Input: part model. Units: mm. Frame: model coordinates. A direction names the side the tool comes from. Coordinates: 2 decimals unless noted, no trailing zeros. Write each loop counter-clockwise with the first axis right and the second up, starting at its lowest first coordinate (ties: lowest second). Pieces come first, ordered by that corner, then holes. Notation, with made-up numbers: (66.5, -24.75) - (125.5, -24.75) arc R32 ccw to (125.5, 3.25) - close; hole circle Ø1 at (16, -32.5). An arc over 180 degrees is marked (long way). Use a Markdown table: item, result. Add a question column.
Q1. Material intervals for probe 1 along Y at (x, z) = (-8, -161.5) (3 decimals); probe 2 along X at (y, z) = (4.5, -37.5) (3 decimals); probe 3 along Y at (x, z) = (24.25, 190.5) (3 decimals), sorted ascending. Write a range as from..to.
Q2. Mould query, pull axis X, two halves, no side actions, for faces 1 (the face through (0, -9.525, -5)), 2 (the face through (-25.4, 0, -5)), 3 (the face through (0, 10, 330.2)). Classes: released by +X, released by -X, zero draft, split by the parting line, or undercut.
Q3. Set-up query: faces 4 (the face through (0, -12.7, -5)), 5 (the face through (-23.79, 1.907, -152.107)), 6 (the face through (22.225, 0, -5)). Return all of +Z, -Z, +X, -X, +Y, -Y with unobstructed straight access to the full face (end or side cutting, diameter ignored); none if empty.
Q4. Section query A-A (z = 1.5). Return the cut outline in (x, y) (3 decimals).
Q5. Pin query (flat end, axial travel): P1, Ø5.5, axis at y = 0, z = -215.9, coming from the -X side. Return the tip coordinate at first contact, or that it passes through.
Q6. Section query B-B (z = 120.65). Return the cut outline in (x, y) (3 decimals).
from build123d import *

# Parameters (mm, degrees)
BOSS_EXTRUDE1_DEPTH              = 330.2
BOSS_EXTRUDE1_DEPTH_BACK         = 330.2
SKETCH3_W                        = 50.8
SKETCH3_H                        = 25.4
SKETCH3_W_2                      = 44.45
SKETCH3_H_2                      = 19.05
F_1_4_0_25_DIAMETER_HOLE3_D      = 6.35
F_1_4_0_25_DIAMETER_HOLE4_D      = 6.35
F_1_4_0_25_DIAMETER_HOLE5_D      = 6.35
F_1_4_0_25_DIAMETER_HOLE6_D      = 6.35
F_1_4_0_25_DIAMETER_HOLE7_D      = 6.35
F_1_4_0_25_DIAMETER_HOLE8_D      = 6.35
F_13_64_0_20313_DIAMETER_HOLE1_D = 5.159502
F_1_2_0_5_DIAMETER_HOLE1_D       = 12.7
F_1_2_0_5_DIAMETER_HOLE1_DEPTH   = 6.35
F_1_2_0_5_DIAMETER_HOLE1_TIP     = 3.815464931


with BuildPart() as part:
    # Sketch3 → Boss-Extrude1 (new, two sides: drawn at the far end of the back side and taken through both)
    with BuildSketch(Plane.XY.offset(-BOSS_EXTRUDE1_DEPTH_BACK)):
        Rectangle(SKETCH3_W, SKETCH3_H)
        Rectangle(SKETCH3_W_2, SKETCH3_H_2, mode=Mode.SUBTRACT)
    extrude(amount=BOSS_EXTRUDE1_DEPTH + BOSS_EXTRUDE1_DEPTH_BACK)

    # 1/4 (0.25) Diameter Hole3 (through all)
    with Locations(Plane.ZY.offset(25.4)):
        with Locations((-317.5, 0)):
            Hole(F_1_4_0_25_DIAMETER_HOLE3_D / 2)

    # 1/4 (0.25) Diameter Hole4 (through all)
    with Locations(Plane.ZY.offset(25.4)):
        with Locations((292.1, 0), (317.5, 0)):
            Hole(F_1_4_0_25_DIAMETER_HOLE4_D / 2)

    # 1/4 (0.25) Diameter Hole5 (through all)
    with Locations(Plane(origin=(25.4, 0, 0), x_dir=(0, 0, -1), z_dir=(1, 0, 0))):
        with Locations((292.1, 0), (266.7, 0)):
            Hole(F_1_4_0_25_DIAMETER_HOLE5_D / 2)

    # 1/4 (0.25) Diameter Hole6 (through all)
    with Locations(Plane(origin=(25.4, 0, 0), x_dir=(0, 0, -1), z_dir=(1, 0, 0))):
        with Locations((215.9, 0), (241.3, 0)):
            Hole(F_1_4_0_25_DIAMETER_HOLE6_D / 2)

    # 1/4 (0.25) Diameter Hole7 (through all)
    with Locations(Plane(origin=(25.4, 0, 0), x_dir=(0, 0, -1), z_dir=(1, 0, 0))):
        with Locations((-190.5, 0), (-215.9, 0)):
            Hole(F_1_4_0_25_DIAMETER_HOLE7_D / 2)

    # 1/4 (0.25) Diameter Hole8 (through all)
    with Locations(Plane(origin=(25.4, 0, 0), x_dir=(0, 0, -1), z_dir=(1, 0, 0))):
        with Locations((-266.7, 0), (-241.3, 0)):
            Hole(F_1_4_0_25_DIAMETER_HOLE8_D / 2)

    # 13/64 (0.20313) Diameter Hole1 (through all)
    with Locations(Plane(origin=(25.4, 0, 0), x_dir=(0, 0, -1), z_dir=(1, 0, 0))):
        with Locations((-152.4, 0), (177.8, 0)):
            Hole(F_13_64_0_20313_DIAMETER_HOLE1_D / 2)

    # 1/2 (0.5) Diameter Hole1
    with Locations(Plane.ZY.offset(25.4)):
        with Locations((-146.050000508, 4.9e-08), (120.65, 1.7e-08)):
            Hole(F_1_2_0_5_DIAMETER_HOLE1_D / 2, depth=F_1_2_0_5_DIAMETER_HOLE1_DEPTH)
            with Locations((0, 0, -(F_1_2_0_5_DIAMETER_HOLE1_DEPTH + F_1_2_0_5_DIAMETER_HOLE1_TIP / 2))):  # 118° drill point
                Cone(0, F_1_2_0_5_DIAMETER_HOLE1_D / 2, F_1_2_0_5_DIAMETER_HOLE1_TIP, mode=Mode.SUBTRACT)


solid = part.part
Values follow:
| question | item | result |
|---|---|---|
| 1 | probe 1 | -12.7..-9.525, 9.525..12.7 |
| 1 | probe 2 | -25.4..-22.225, 22.225..25.4 |
| 1 | probe 3 | -12.7..-3.175, 3.175..12.7 |
| 2 | face 1 | undercut |
| 2 | face 2 | released by -X |
| 2 | face 3 | zero draft |
| 3 | face 4 | +Z, -Z, +X, -X, -Y |
| 3 | face 5 | -X |
| 3 | face 6 | +Z, -Z |
| 4 | outline | (-25.4, -12.7) - (25.4, -12.7) - (25.4, 12.7) - (-25.4, 12.7) - close; hole (-22.225, -9.525) - (22.225, -9.525) - (22.225, 9.525) - (-22.225, 9.525) - close |
| 5 | P1 | through |
| 6 | outline | (-25.4, -12.7) - (25.4, -12.7) - (25.4, 12.7) - (-25.4, 12.7) - (-25.4, 6.35) - (-22.225, 6.35) - (-22.225, 9.525) - (22.225, 9.525) - (22.225, -9.525) - (-22.225, -9.525) - (-22.225, -6.35) - (-25.4, -6.35) - close |
